Autodesk Inventor part; units mm, degrees
ref_plane "YZ Plane" through (0, 0, 0) normal (1, 0, 0) x (0, 1, 0)
ref_plane "XZ Plane" through (0, 0, 0) normal (0, 1, 0) x (-1, 0, 0)
ref_plane "XY Plane" through (0, 0, 0) normal (0, 0, 1) x (1, 0, 0)
sketch "Boceto1" plane through (0, 0, 0) normal (0, 0, 1) x (1, 0, 0)
  line L0 (0.5, -3) -> (-0.5, -3)
  line L1 (-0.5, -3) -> (-0.5, 3)
  line L2 (-0.5, 3) -> (0.5, 3)
  line L3 (0.5, 3) -> (0.5, -3)
  line L4 (0.5, -3) -> (-0.5, 3) construction
  line L5 (-0.5, -3) -> (0.5, 3) construction
  point P0 (0, 0)
  dimension "d0" = 1
  dimension "d1" = 6
sketch "Boceto2" plane through (0, 0, 0) normal (1, 0, 0) x (0, 1, 0)
  line L0 (0, 0) -> (0, 7)
  line L1 (2.5, 1.1547) -> (2.5, 6.2702)
  line L2 (2.5, 6.2702) -> (2.0787, 7)
  line L3 (2.0787, 7) -> (0, 7)
  line L4 (2.5, 1.1547) -> (2.6776, 1.1547)
  line L5 (2.6776, 1.1547) -> (2.7854, 1.1547)
  line L6 (2.7854, 1.1547) -> (2.7854, 0.1547)
  line L7 (2.7854, 0.1547) -> (3.1939, 0.4965)
  line L8 (3.1939, 0.4965) -> (3.3939, 0.4965)
  line L9 (3.3939, 0.4965) -> (3, 0)
  line L10 (-2.5, 1.1547) -> (-2.5, 6.2702)
  line L11 (-2.5, 6.2702) -> (-2.0787, 7)
  line L12 (-2.0787, 7) -> (0, 7)
  line L13 (-2.5, 1.1547) -> (-2.6776, 1.1547)
  line L14 (-2.6776, 1.1547) -> (-2.7854, 1.1547)
  line L15 (-2.7854, 1.1547) -> (-2.7854, 0.1547)
  line L16 (-2.7854, 0.1547) -> (-3.1939, 0.4965)
  line L17 (-3.1939, 0.4965) -> (-3.3939, 0.4965)
  line L18 (-3.3939, 0.4965) -> (-3, 0)
  line L19 (3, 0) -> (-3, 0)
  circle A0 centre (0, 5) radius 1
  dimension "d2" = 7
  dimension "d3" = 120
  dimension "d8" = 0.2
  dimension "d9" = 1
  dimension "d10" = 2
  dimension "d11" = 2
extrude "Extrusión1" add sketch "Boceto2" along normal mid plane 1 contours L19 L18 L17 L16 L15 L14 L13 L10 L11 L12 L0 A0 | L0 A0 L3 L2 L1 L4 L5 L6 L7 L8 L9 L19
extrude "Extrusión2" add sketch "Boceto1" against normal blind 1
sketch "Boceto3" plane through (0, 0, -1) normal (0, 0, -1) x (-1, 0, 0)
  line L0 (-0.5, 4) -> (0.5, 4)
  line L1 (0.5, 4) -> (0.5, -4)
  line L2 (0.5, -4) -> (-0.5, -4)
  line L3 (-0.5, -4) -> (-0.5, 4)
  line L4 (-0.5, 4) -> (0.5, -4) construction
  line L5 (0.5, 4) -> (-0.5, -4) construction
  line L6 (-0.5, 2) -> (0.5, 2)
  line L7 (0.5, 2) -> (0.5, -2)
  line L8 (0.5, -2) -> (-0.5, -2)
  line L9 (-0.5, -2) -> (-0.5, 2)
  line L10 (-0.5, 2) -> (0.5, -2) construction
  line L11 (0.5, 2) -> (-0.5, -2) construction
  point P0 (0, 0)
  dimension "d16" = 8
  dimension "d17" = 4
extrude "Extrusión3" add sketch "Boceto3" along normal blind 4 contours L0 L1 L6 L3 | L8 L1 L2 L3
sketch "Boceto4" plane through (0, 0, -1) normal (0, 0, -1) x (-1, 0, 0)
  line L0 (-0.5, 2) -> (0.5, 2)
  line L1 (0.5, 2) -> (0.5, -2)
  line L2 (0.5, -2) -> (-0.5, -2)
  line L3 (-0.5, -2) -> (-0.5, 2)
  line L4 (-0.5, 2) -> (0.5, -2) construction
  line L5 (0.5, 2) -> (-0.5, -2) construction
  point P0 (0, 0)
  dimension "d20" = 1
  dimension "d21" = 4
extrude "Extrusión4" add sketch "Boceto4" along normal blind 1
properties part number "Polo2"
Verification items for the finished model (mm, model axes). A direction names the side the tool comes from. Give positions to 0.01 mm unless a question says otherwise; leave off trailing zeros. Loops run counter-clockwise (first coordinate to the right, second up) from the corner with the lowest first, then second, coordinate; pieces in that order, holes last.
1) Set-up check for faces 5 (the flat face through (0, 2.785, 1)), 6 (the flat face through (0, 0, -2)), 7 (the flat face through (0, -3, -0.5)), 8 (the flat face through (0, 3, -0.5)), 9 (the flat face through (0, 2.5, 4)): record each of +Z, -Z, +X, -X, +Y, -Y from which the full face is reachable in a straight line by a thin tool's end or side.
2) Sectioned sample at B-B, the plane z = -3.5. Enter the section's corners in (x, y), then the cut area to 3 significant figures.
3) Depth check by flat-ended pin: pin 1 Ø0.5 at (x, z) = (0, 1) entering from -Y; pin 2 Ø0.5 at (x, z) = (0, -0.5) entering from -Y; pin 3 Ø1.5 at (y, z) = (-0.5, 5.5) entering from +X. Enter the tip coordinate at first touch or a pass-through.
4) Sectioned sample at A-A, the plane y = 0. Enter the section's corners in (x, z).
5) Sectioned sample at C-C, the plane x = 0.05. Enter the section's corners in (y, z).
6) Draft check along Z on faces 1 (the flat face through (0, -2.785, 1)), 2 (the flat face through (0, 0, 7)), 3 (the flat face through (0, -3.5, -1)), 4 (the flat face through (0, -3, -5)). Enter one of: pulls with the +Z half, pulls with the -Z half, needs draft (parallel to the pull), parting line crosses it, or undercut.
7) Thickness scan on line 1 along Y through (x, z) = (0, 5); line 2 along Y through (x, z) = (-0.05, -3.5); line 3 along Z through (x, y) = (-0.05, 0). Record the ranges inside material, lowest first.
Answers:
1. face 5: +Z, +X, -X
1. face 6: -Z, +X, -X
1. face 7: +X, -X, -Y
1. face 8: +X, -X, +Y
1. face 9: +Z, +X, -X, +Y
2. outline: (-0.5, -4) - (0.5, -4) - (0.5, -2) - (-0.5, -2) - close; (-0.5, 2) - (0.5, 2) - (0.5, 4) - (-0.5, 4) - close
2. area: 4.00 mm2
3. pin 1: stops at y = -2.79
3. pin 2: stops at y = -3
3. pin 3: stops at x = 0.5
4. outline: (-0.5, -2) - (0.5, -2) - (0.5, 4) - (-0.5, 4) - close; (-0.5, 6) - (0.5, 6) - (0.5, 7) - (-0.5, 7) - close
5. outline: (-4, -5) - (-2, -5) - (-2, -2) - (2, -2) - (2, -5) - (4, -5) - (4, -1) - (3, -1) - (3, 0) - (3.39, 0.5) - (3.19, 0.5) - (2.79, 0.15) - (2.79, 1.15) - (2.5, 1.15) - (2.5, 6.27) - (2.08, 7) - (-2.08, 7) - (-2.5, 6.27) - (-2.5, 1.15) - (-2.79, 1.15) - (-2.79, 0.15) - (-3.19, 0.5) - (-3.39, 0.5) - (-3, 0) - (-3, -1) - (-4, -1) - close; hole circle Ø2 at (0, 5)
6. face 1: needs draft
6. face 2: pulls with the +Z half
6. face 3: undercut
6. face 4: pulls with the -Z half
7. line 1: y = -2.5 to -1, 1 to 2.5
7. line 2: y = -4 to -2, 2 to 4
7. line 3: z = -2 to 4, 6 to 7
